from build123d import *

# Parameters (mm, degrees)
F0_R     = 2.55
F1_DEPTH = 30
F2_R     = 12.7
F2_R_2   = 10.5
F3_DEPTH = 20
F4_DEPTH = 25


with BuildPart() as f1:
    # F0 (on Front) → F1 (new body)
    with BuildSketch(Plane.XZ):
        with BuildLine():
            ThreePointArc((0, 5), (1.4644660941, 1.4644660941), (5, 0))
            Line((5, 0), (115, 0))
            ThreePointArc((115, 0), (118.5355339059, 1.4644660941), (120, 5))
            Line((120, 5), (120, 115))
            ThreePointArc((120, 115), (118.5355339059, 118.5355339059), (115, 120))
            Line((115, 120), (5, 120))
            ThreePointArc((5, 120), (1.4644660941, 118.5355339059), (0, 115))
            Line((0, 115), (0, 5))
        make_face()
        with Locations((7.5, 7.5)):
            Circle(F0_R, mode=Mode.SUBTRACT)
        with Locations((112.5, 7.5)):
            Circle(F0_R, mode=Mode.SUBTRACT)
        with BuildLine():
            Line((4, 101.8933982822), (7.5, 101.8933982822))
            ThreePointArc((7.5, 101.8933982822), (15, 105), (18.1066017178, 112.5))
            Line((18.1066017178, 112.5), (18.1066017178, 116))
            Line((18.1066017178, 116), (101.8933982822, 116))
            Line((101.8933982822, 116), (101.8933982822, 112.5))
            ThreePointArc((101.8933982822, 112.5), (105, 105), (112.5, 101.8933982822))
            Line((112.5, 101.8933982822), (116, 101.8933982822))
            Line((116, 101.8933982822), (116, 18.1066017178))
            Line((116, 18.1066017178), (112.5, 18.1066017178))
            ThreePointArc((112.5, 18.1066017178), (105, 15), (101.8933982822, 7.5))
            Line((101.8933982822, 7.5), (101.8933982822, 4))
            Line((101.8933982822, 4), (18.1066017178, 4))
            Line((18.1066017178, 4), (18.1066017178, 7.5))
            ThreePointArc((18.1066017178, 7.5), (15, 15), (7.5, 18.1066017178))
            Line((7.5, 18.1066017178), (4, 18.1066017178))
            Line((4, 18.1066017178), (4, 101.8933982822))
        make_face(mode=Mode.SUBTRACT)
        with Locations((7.5, 112.5)):
            Circle(F0_R, mode=Mode.SUBTRACT)
        with Locations((112.5, 112.5)):
            Circle(F0_R, mode=Mode.SUBTRACT)
    extrude(amount=F1_DEPTH)

    # F2 (on face) → F3 (join)
    with BuildSketch(Plane.XY.offset(120)):
        with Locations((30, -15)):
            Circle(F2_R)
        with Locations((30, -15)):
            Circle(F2_R_2, mode=Mode.SUBTRACT)
    extrude(amount=F3_DEPTH)

    # F4 (cut): a face of the model
    f4_faces = [f1.faces().sort_by_distance(p)[0] for p in [
        (30, -15, 120),
    ]]
    extrude(f4_faces, amount=-F4_DEPTH, mode=Mode.SUBTRACT)


solid = f1.part
Check sheet for the modelled part. Datum: model origin and axes. Units: mm. A direction names the side the tool comes from. Round coordinates to 2 decimals unless told otherwise and drop trailing zeros. Loops run counter-clockwise (first coordinate to the right, second up) from the corner with the lowest first, then second, coordinate; pieces in that order, holes last.
1. Scan lines: probe 1 along Z at (x, y) = (7.5, -13); probe 2 along Z at (x, y) = (79, -17.25). Record each from-to range of solid material in increasing order.
2. Gauge pin test, flat end, axial feed: pin 1 Ø1 at (x, y) = (114, -20) entering from +Z. Record the tip position at first contact, or that the pin passes through.
3. Sectioned sample at A-A on z = 98.5. Record the boundary of the cut face in (x, y).
4. Sectioned sample at D-D on y = -15. Give the number of separate pieces and of enclosed holes in the cut face, and give its area (3 significant figures).
5. Mould release check, pull along Z, two halves, no side actions. Record for faces 1 (the flat face through (60, 0, 118)), 2 (the cylindrical face through (105, -15, 105)), 3 (the cylindrical face through (2, -15, 119)): released by +Z, released by -Z, zero draft, split by the parting line, or undercut.
6. Set-up check for faces 4 (the flat face through (0, -15, 61)), 5 (the flat face through (69, -15, 116)), 6 (the cylindrical face through (42.114, -11.185, 129.86)): record each of +Z, -Z, +X, -X, +Y, -Y from which the full face is reachable in a straight line by a thin tool's end or side.
7. Sectioned sample at B-B on x = 30. Record the boundary of the cut face in (y, z).
8. Sectioned sample at C-C on x = 91. Record the boundary of the cut face in (y, z), and give its area (3 significant figures).
Recorded:
1. probe 1: z = 0 to 4.95, 10.05 to 18.11, 101.89 to 109.95, 115.05 to 120
1. probe 2: z = 0 to 4, 116 to 120
2. pin 1: stops at z = 120
3. outline: (0, -30) - (4, -30) - (4, 0) - (0, 0) - close; (116, -30) - (120, -30) - (120, 0) - (116, 0) - close
4. separate pieces: 1
4. enclosed holes: 4
4. area: 2,460 mm2
5. face 1: zero draft
5. face 2: undercut
5. face 3: released by +Z
6. face 4: +Z, -Z, -X, +Y, -Y
6. face 5: +Y, -Y
6. face 6: +Z
7. outline: (-30, 0) - (0, 0) - (0, 4) - (-30, 4) - close; (-30, 116) - (-25.5, 116) - (-25.5, 140) - (-27.7, 140) - (-27.7, 120) - (-30, 120) - close; (-4.5, 116) - (0, 116) - (0, 120) - (-2.3, 120) - (-2.3, 140) - (-4.5, 140) - close
8. outline: (-30, 0) - (0, 0) - (0, 4) - (-30, 4) - close; (-30, 116) - (0, 116) - (0, 120) - (-30, 120) - close
8. area: 240 mm2
